Design review of the part built by this model. Coordinates are the model's own, in mm. A direction names the side the tool comes from. Coordinates: 2 decimals unless noted, no trailing zeros. Write each loop counter-clockwise with the first axis right and the second up, starting at its lowest first coordinate (ties: lowest second). Pieces come first, ordered by that corner, then holes. Notation, with made-up numbers: M 28.25,3 L 62.25,3 A24 ccw 62.25,13 Z; hole C -21,43 d5. An arc over 180 degrees is marked long. Write item = value, one per line.
```python
from build123d import *

# Parameters (mm, degrees)
F1_DEPTH = 12
F2_R     = 4
F3_DEPTH = 10
F4_R     = 3.25
F5_DEPTH = 21.001


with BuildPart() as f1:
    # F0 (on Front) → F1 (new body)
    with BuildSketch(Plane.XZ):
        Polygon((-15, 0), (0, 0), (15, 0), (15, -10), (25, -10), (25, 11), (0, 11), (-25, 11), (-25, -10), (-15, -10), align=None)
    extrude(amount=F1_DEPTH)

    # F2 (on face) → F3 (cut)
    with BuildSketch(Plane.YZ.offset(25)):
        with Locations((-6, 5)):
            Circle(F2_R)
    extrude(amount=-F3_DEPTH, mode=Mode.SUBTRACT)

    # F4 (on face) → F5 (cut, through all)
    with BuildSketch(Plane.XY.offset(11)):
        with Locations((0, -6)):
            Circle(F4_R)
    extrude(amount=-F5_DEPTH, mode=Mode.SUBTRACT)


solid = f1.part
```
Q1. For P1, Ø6, axis at x = 0, y = -6, coming from the -Z side, flat-tipped, find the tip position at first contact; note if it passes through.
Check result:
P1 = through
Q2. Machinability: for faces 1 (the flat face through (-25, -6, 1)), 2 (the flat face through (15, -6, -5)), 3 (the cylindrical face through (20.07, -6.867, 1.095)), which of the approach directions +Z, -Z, +X, -X, +Y, -Y give a long, thin tool a straight path to every point of the face, cutting with its end or side? Answer none if there is none.
Check result:
face_1 = +Z, -Z, -X, +Y, -Y
face_2 = -Z, +Y, -Y
face_3 = +X
Q3. Consider section B-B, the plane x = 0. State the section outline as (y, z) points.
Check result:
outline = M -12,0 L -9.25,0 L -9.25,11 L -12,11 Z; M -2.75,0 L 0,0 L 0,11 L -2.75,11 Z
Q4. The part is to be moulded in two halves that separate along X. For faces 4 (the flat face through (15, -6, 5)), 5 (the flat face through (-4, -6, 0)), 6 (the flat face through (-20, -6, -10)), say which applies: +X half, -X half, draft (parallel to the pull), parting line (faces both ways), or undercut.
Check result:
face_4 = +X half
face_5 = undercut
face_6 = draft
Q5. Consider section C-C, the plane y = -6. State the section outline as (x, z) points.
Check result:
outline = M -25,-10 L -15,-10 L -15,0 L -3.25,0 L -3.25,11 L -25,11 Z; M 3.25,0 L 15,0 L 15,-10 L 25,-10 L 25,1 L 15,1 L 15,9 L 25,9 L 25,11 L 3.25,11 Z
Q6. Wall thickness on line 1 (X direction, y = -11.5, z = -4.5); line 2 (Z direction, x = 19.5, y = -6); line 3 (Z direction, x = -5, y = -3.5): over which ranges is each line inside the solid? List them lowest first.
Check result:
line_1 = -25 to -15, 15 to 25
line_2 = -10 to 1, 9 to 11
line_3 = 0 to 11
Q7. Consider section D-D, the plane z = -1. State the section outline as (x, y) points, and give its area (3 significant figures).
Check result:
outline = M -25,-12 L -15,-12 L -15,0 L -25,0 Z; M 15,-12 L 25,-12 L 25,0 L 15,0 Z
area = 240 mm²
Q8. Consider section A-A, the plane z = 5. State the section outline as (x, y) points, and give its area (3 significant figures).
Check result:
outline = M -25,-12 L 25,-12 L 25,-10 L 15,-10 L 15,-2 L 25,-2 L 25,0 L -25,0 Z; hole C 0,-6 d6.5
area = 487 mm²
